from build123d import *

# Parameters (mm, degrees)
F1_DEPTH = 1.4
F2_W     = 1
F2_H     = 2
F3_DEPTH = 0.1
F4_W     = 0.5
F4_H     = 0.15
F5_DEPTH = 4


with BuildPart() as f1:
    # F0 (on Top) → F1 (new body)
    with BuildSketch(Plane.XY):
        Polygon((1.6, -1.35), (1.6, 1.35), (-0.9672628953, 1.35), (-1.6, 0.628211031), (-1.6, -1.35), align=None)
    extrude(amount=F1_DEPTH)

    # F2 (on face) → F3 (cut)
    with BuildSketch(Plane.XY.offset(1.4)):
        with Locations((0.83, 0)):
            Rectangle(F2_W, F2_H)
        Polygon((-0.33, -1), (-0.33, 1), (-0.8539721624, 1), (-1.33, 0.4569756704), (-1.33, -1), align=None)
    extrude(amount=-F3_DEPTH, mode=Mode.SUBTRACT)

    # F6: F5 across plane


with BuildPart() as f5:
    # F4 (on Front) → F5 (new body)
    with BuildSketch(Plane.XZ):
        with Locations((-0.9, 0.475)):
            Rectangle(F4_W, F4_H)
    extrude(amount=F5_DEPTH)


with BuildPart() as f1_1:
    add(f1.part)
    add(f5.part.mirror(Plane.YZ))



with BuildPart() as f9:
    # F9: sweep along a path in F8
    with BuildLine(Plane.YZ.offset(-0.9)) as f9_path:
        Line((0, 0.475), (2.35, 0.475))
        ThreePointArc((2.35, 0.475), (2.7035533906, 0.3285533906), (2.85, -0.025))
        Line((2.85, -0.025), (2.85, -1.025))
        ThreePointArc((2.85, -1.025), (2.7035533906, -1.3785533906), (2.35, -1.525))
        Line((2.35, -1.525), (-4, -1.525))
    # F4 (on Front) → F9 (sweep)
    with BuildSketch(Plane.XZ):
        with Locations((-0.9, 0.475)):
            Rectangle(F4_W, F4_H)
    sweep(path=f9_path.line)


with BuildPart() as f1_2:
    add(f1_1.part)

    add(f5.part)  # F10 merges F5

    add(f9.part)  # F10 merges F9
    # F10: F9 across plane
    add(f9.part.mirror(Plane.YZ))


solid = f1_2.part
Work out the finished part from the listing and answer in its coordinate system (mm). A direction names the side the tool comes from. Give positions to 0.01 mm unless a question says otherwise; leave off trailing zeros. Order: outer loops, then holes, each group sorted by start corner. A loop starts at its lowest first (then second) coordinate and runs counter-clockwise, first axis right, second up. Notation, with made-up numbers: (42, 88.5) - (97, 88.5) arc R26 cw to (97, 102.5) - close; hole circle Ø8 at (9.25, 67.25). An arc over 180 degrees is marked (long way). Answer as CSV lines item,"result". Start each with the question number.
Q1. Find the intervals of material crossed by L1, parallel to Z at x = -0.9, y = -0.5; L2, parallel to X at y = 1.75, z = 0.5; L3, parallel to Z at x = -1, y = 1, in increasing order. Write a range as [from, to].
Q2. The part is cut by section D-D (z = 0.1). Write down the section's boundary in (x, y), then the cut area to 3 significant figures.
Q3. The mould has two halves that part along Y. Classify faces 4 (the face through (1, 0, 1.3)), 5 (the face through (0, 0, 1.4)): +Y half, -Y half, draft (parallel to the pull), parting line (faces both ways), or undercut.
Q4. The part is cut by section A-A (y = -3). Write down the section's boundary in (x, z).
Q5. The part is cut by section C-C (y = 0.75). Write down the section's boundary in (x, z).
Q6. The part is cut by section B-B (z = -0.25). Write down the section's boundary in (x, y) (3 decimals), then the cut area to 3 significant figures.
Q7. Given pin 1 Ø0.5 at (x, y) = (1, -2.5) entering from +Z, flat-ended and moving along its own axis, determine where the tip first touches the part or whether it passes through.
Q8. For faces 1 (the face through (-1.6, 0, 1)), 2 (the face through (-1, 0, 1.3)), 3 (the face through (0, 0, 0)), determine the directions among +Z, -Z, +X, -X, +Y, -Y from which every point of the face is accessible in a straight line to the end or side of a thin tool.
Check result:
1,L1,"z = [-1.6, -1.45], [0, 1.3]"
1,L2,"x = [-1.15, -0.65], [0.65, 1.15]"
1,L3,"z = [-1.6, -1.45], [0, 1.4]"
2,outline,"(-1.6, -1.35) - (1.6, -1.35) - (1.6, 1.35) - (-0.97, 1.35) - (-1.6, 0.63) - close; (-1.15, 2.76) - (-0.65, 2.76) - (-0.65, 2.91) - (-1.15, 2.91) - close; (0.65, 2.76) - (1.15, 2.76) - (1.15, 2.91) - (0.65, 2.91) - close"
2,area,"8.57 mm²"
3,face 4,"undercut"
3,face 5,"draft"
4,outline,"(-1.15, -1.6) - (-0.65, -1.6) - (-0.65, -1.45) - (-1.15, -1.45) - close; (-1.15, 0.4) - (-0.65, 0.4) - (-0.65, 0.55) - (-1.15, 0.55) - close; (0.65, -1.6) - (1.15, -1.6) - (1.15, -1.45) - (0.65, -1.45) - close; (0.65, 0.4) - (1.15, 0.4) - (1.15, 0.55) - (0.65, 0.55) - close"
5,outline,"(-1.49, 0) - (1.6, 0) - (1.6, 1.4) - (1.33, 1.4) - (1.33, 1.3) - (0.33, 1.3) - (0.33, 1.4) - (-0.33, 1.4) - (-0.33, 1.3) - (-1.07, 1.3) - (-1.07, 1.4) - (-1.49, 1.4) - close; (-1.15, -1.6) - (-0.65, -1.6) - (-0.65, -1.45) - (-1.15, -1.45) - close; (0.65, -1.6) - (1.15, -1.6) - (1.15, -1.45) - (0.65, -1.45) - close"
6,outline,"(-1.15, 2.775) - (-0.65, 2.775) - (-0.65, 2.925) - (-1.15, 2.925) - close; (0.65, 2.775) - (1.15, 2.775) - (1.15, 2.925) - (0.65, 2.925) - close"
6,area,"0.150 mm²"
7,pin 1,"stops at z = 0.55"
8,face 1,"+Z, -Z, -X, +Y, -Y"
8,face 2,"+Z"
8,face 3,"+X, -X, -Y"
